The listing builds one solid part. Answer for the finished solid, in the listing's coordinates (mm). Give positions to 0.01 mm unless a question says otherwise; leave off trailing zeros. Write each loop counter-clockwise with the first axis right and the second up, starting at its lowest first coordinate (ties: lowest second). Pieces come first, ordered by that corner, then holes. Notation, with made-up numbers: (28, 23) - (81, 23) arc R29 ccw to (81, 57) - close; hole circle Ø9 at (68, 81.5). An arc over 180 degrees is marked (long way). One line per item, written item: value. Start each with the question number.
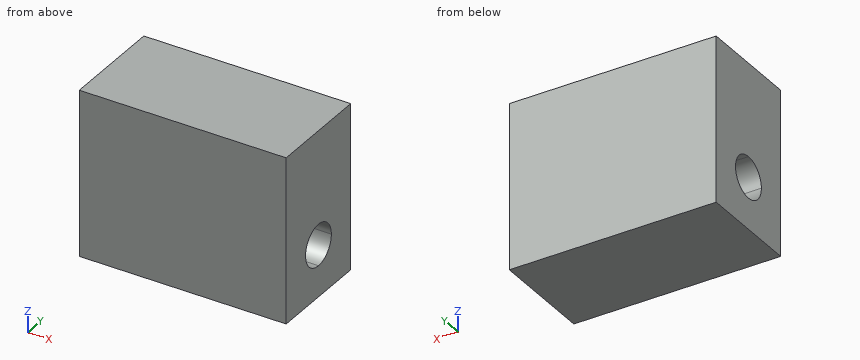
from build123d import *

# Parameters (mm, degrees)
F1_DEPTH = 25.4


with BuildPart() as f1:
    # F0 (on Right) → F1 (new body)
    with BuildSketch(Plane.YZ):
        with BuildLine():
            Line((0, -13.97), (0, 0))
            Line((0, 0), (-6.35, 0))
            Line((-6.35, 0), (-6.35, -11.43))
            ThreePointArc((-6.35, -11.43), (-4.553949, -12.173949), (-3.81, -13.97))
            Line((-3.81, -13.97), (0, -13.97))
        make_face()
        with BuildLine():
            Line((-6.35, -11.43), (-6.35, 0))
            Line((-6.35, 0), (-12.7, 0))
            Line((-12.7, 0), (-12.7, -13.97))
            Line((-12.7, -13.97), (-8.89, -13.97))
            ThreePointArc((-8.89, -13.97), (-8.146051, -12.173949), (-6.35, -11.43))
        make_face()
        with BuildLine():
            Line((-8.89, -13.97), (-12.7, -13.97))
            Line((-12.7, -13.97), (-12.7, -20.32))
            Line((-12.7, -20.32), (-6.35, -20.32))
            Line((-6.35, -20.32), (-6.35, -16.51))
            ThreePointArc((-6.35, -16.51), (-8.146051, -15.766051), (-8.89, -13.97))
        make_face()
        with BuildLine():
            Line((0, -20.32), (0, -13.97))
            Line((0, -13.97), (-3.81, -13.97))
            ThreePointArc((-3.81, -13.97), (-4.553949, -15.766051), (-6.35, -16.51))
            Line((-6.35, -16.51), (-6.35, -20.32))
            Line((-6.35, -20.32), (0, -20.32))
        make_face()
    extrude(amount=F1_DEPTH)


solid = f1.part
Item 1: Find section A-A on x = 14. Determine the outline of the cut face in (y, z).
Item 2: This flat-tipped pin is pushed along its axis until it touches: pin 1 Ø3 at (x, z) = (9, -4.5) entering from +Y. Where does it stop, or does it pass through?
Item 3: Find section B-B on y = -5.25. Determine the outline of the cut face in (x, z).
Item 4: Straight lines are drawn through the part: line 1 along Z through (x, y) = (20.5, -5.25); line 2 along Z through (x, y) = (17.5, -5); line 3 along Y through (x, z) = (15.25, -11.75). For each, find the intervals that lie inside material, in ascending order.
Item 5: Find section C-C on z = -15.25. Determine the outline of the cut face in (x, y), plus the area to 3 significant figures.
Values:
1. outline: (-12.7, -20.32) - (0, -20.32) - (0, 0) - (-12.7, 0) - close; hole (-8.89, -13.97) arc R2.54 ccw to (-6.35, -16.51) arc R2.54 ccw to (-3.81, -13.97) arc R2.54 ccw to (-6.35, -11.43) arc R2.54 ccw to start
2. pin 1: y = 0
3. outline: (0, -20.32) - (25.4, -20.32) - (25.4, -16.26) - (0, -16.26) - close; (0, -11.68) - (25.4, -11.68) - (25.4, 0) - (0, 0) - close
4. line 1: -20.32 to -16.26, -11.68 to 0
4. line 2: -20.32 to -16.12, -11.82 to 0
4. line 3: -12.7 to -7.58, -5.12 to 0
5. outline: (0, -12.7) - (25.4, -12.7) - (25.4, -8.54) - (0, -8.54) - close; (0, -4.16) - (25.4, -4.16) - (25.4, 0) - (0, 0) - close
5. area: 211 mm^2
